Autodesk Inventor part; units mm, degrees
ref_plane "YZ Plane" through (0, 0, 0) normal (1, 0, 0) x (0, 1, 0)
ref_plane "XZ Plane" through (0, 0, 0) normal (0, 1, 0) x (-1, 0, 0)
ref_plane "XY Plane" through (0, 0, 0) normal (0, 0, 1) x (1, 0, 0)
sketch "Sketch1" plane through (0, 0, 0) normal (0, 0, 1) x (1, 0, 0)
  line L0 (-19.7993, 68.1553) -> (17.5761, 68.1553)
  line L1 (20.5597, 66.0662) -> (62.3445, -48.7367)
  line L2 (-19.7993, 68.1553) -> (-19.7993, -48.7367)
  line L3 (-19.7993, -48.7367) -> (62.3445, -48.7367)
  arc A0 (20.5597, 66.0662) -> (17.5761, 68.1553) centre (17.5761, 64.9803) ccw
  point P0 (0, 0)
  point P1 (19.7993, 68.1553)
  dimension "d0" = 110
  dimension "d1" = 39.5986
  dimension "d2" = 3.175
  dimension "d3" = 122.1707
extrude "Extrusion1" add sketch "Sketch1" along normal blind 63.5
sketch "Sketch2" plane through (-19.7993, -48.7367, 0) normal (-1, 0, 0) x (0, 0, 1)
  line L0 (10.7282, 97.9332) -> (52.7214, 97.9332)
  line L1 (52.7214, 97.9332) -> (52.7214, 3.0652)
  line L2 (52.7214, 3.0652) -> (10.7282, 3.0652)
  line L3 (10.7282, 3.0652) -> (10.7282, 97.9332)
  point P0 (0, 48.7367)
extrude "Extrusion2" cut sketch "Sketch2" against normal blind 34.925
move faces "Move1" translate (0, 0, -6.35) faces at (21.035, -10.4691, 63.5)
move faces "Move2" translate (0, 0, 4.7752) faces at (21.035, -10.4691, 0)
move faces "Move3" translate (0, 6.35, 0) faces at (7.582, -48.7367, 22.2335)
move faces "Move4" translate (0, 0, 7.9502) faces at (20.2646, -6.2358, 57.15)
For this review, take the finished solid that the model builds, in its own axes (mm). A direction names the side the tool comes from. Give positions to 0.01 mm unless a question says otherwise; leave off trailing zeros. Order: outer loops, then holes, each group sorted by start corner. A loop starts at its lowest first (then second) coordinate and runs counter-clockwise, first axis right, second up. Notation, with made-up numbers: (76, 60.5) - (111, 60.5) arc R31 cw to (111, 94.5) - close; hole circle Ø10 at (28.5, 44.25). An arc over 180 degrees is marked (long way). Answer as a JSON object with one key per item and string values. Group by question number.
Item 1: Take a section at D-D on x = 22. Give the boundary of the cut face in (y, z).
Item 2: Machinability: for faces 5 (the flat face through (-3, 3, 10.728)), 6 (the flat face through (40.02, 12.6, 34.52)), which of the approach directions +Z, -Z, +X, -X, +Y, -Y give a long, thin tool a straight path to every point of the face, cutting with its end or side? Answer none if there is none.
Item 3: Take a section at C-C on y = -12. Give the boundary of the cut face in (x, z).
Item 4: Clearance check with flat-ended pins moving along their axes: pin 1 Ø5 at (y, z) = (33, 18) entering from +X; pin 2 Ø6 at (y, z) = (21.5, 20.5) entering from -X; pin 3 Ø10.5 at (x, z) = (3, 37) entering from -Y. State where each tip first meets the part, or that it passes through.
Item 5: Take a section at A-A on z = 18. Give the boundary of the cut face in (x, y).
Item 6: Wall thickness on line 1 along Z through (x, y) = (-2, -0.5); line 2 along Y through (x, z) = (8.5, 25.5); line 3 along X through (y, z) = (22.5, 56.5): over which ranges is each line inside the solid? List them lowest first.
Item 7: Take a section at B-B on x = 3. Give the boundary of the cut face in (y, z).
Item 8: Draft analysis for pull direction Z (two halves, no side actions). For faces 1 (the cylindrical face through (19.37, 67.6, 34.52)), 2 (the flat face through (15.126, 4, 31)), 3 (the flat face through (-3, 4, 52.721)), 4 (the flat face through (11, 14, 4.775)), state which applies: pulls with the +Z half, pulls with the -Z half, needs draft (parallel to the pull), parting line crosses it, or undercut.
Reported:
{
 "1": {"outline": "(-42.39, 4.78) - (62.11, 4.78) - (62.11, 65.1) - (-42.39, 65.1) - close"},
 "2": {"face 5": "-X, -Y", "face 6": "+Z, -Z, +X, +Y"},
 "3": {"outline": "(-19.8, 4.78) - (48.97, 4.78) - (48.97, 65.1) - (-19.8, 65.1) - (-19.8, 52.72) - (15.13, 52.72) - (15.13, 10.73) - (-19.8, 10.73) - close"},
 "4": {"pin 1": "x = 33.5", "pin 2": "x = 15.13", "pin 3": "y = 49.2"},
 "5": {"outline": "(-19.8, 49.2) - (15.13, 49.2) - (15.13, -42.39) - (60.03, -42.39) - (20.56, 66.07) arc R3.17 ccw to (17.58, 68.16) - (-19.8, 68.16) - close"},
 "6": {"line 1": "4.78 to 10.73, 52.72 to 65.1", "line 2": "49.2 to 68.16", "line 3": "-19.8 to 36.42"},
 "7": {"outline": "(-42.39, 4.78) - (68.16, 4.78) - (68.16, 65.1) - (-42.39, 65.1) - (-42.39, 52.72) - (49.2, 52.72) - (49.2, 10.73) - (-42.39, 10.73) - close"},
 "8": {"face 1": "needs draft", "face 2": "undercut", "face 3": "undercut", "face 4": "pulls with the -Z half"}
}
